from build123d import *

# Parameters (mm, degrees)
ESQUISSE1_W             = 190
ESQUISSE1_H             = 20
BOSS_EXTRU_1_DEPTH      = 6
ESQUISSE2_W             = 6
ESQUISSE2_H             = 20
ENL_V_MAT_EXTRU_1_DEPTH = 3
ESQUISSE3_R             = 1.5
ENL_V_MAT_EXTRU_2_DEPTH = 6


with BuildPart() as part:
    # Esquisse1 → Boss.-Extru.1 (new body)
    with BuildSketch(Plane.XY):
        Rectangle(ESQUISSE1_W, ESQUISSE1_H)
    extrude(amount=BOSS_EXTRU_1_DEPTH)

    # Esquisse2 → Enlèv. mat.-Extru.1 (cut)
    with BuildSketch(Plane.XY.offset(6)):
        with Locations((-92, 0)):
            Rectangle(ESQUISSE2_W, ESQUISSE2_H)
        with Locations((92, 0)):
            Rectangle(ESQUISSE2_W, ESQUISSE2_H)
    extrude(amount=-ENL_V_MAT_EXTRU_1_DEPTH, mode=Mode.SUBTRACT)

    # Esquisse3 → Enlèv. mat.-Extru.2 (cut)
    with BuildSketch(Plane(origin=(0, 0, 0), x_dir=(-1, 0, 0), z_dir=(0, 0, -1))):
        with Locations((-92, -7)):
            Circle(ESQUISSE3_R)
        with Locations((-92, 7)):
            Circle(ESQUISSE3_R)
        with Locations(Location((92, 7, 0), (0, 0, 180))):
            Circle(ESQUISSE3_R)
        with Locations(Location((92, -7, 0), (0, 0, 180))):
            Circle(ESQUISSE3_R)
    extrude(amount=-ENL_V_MAT_EXTRU_2_DEPTH, mode=Mode.SUBTRACT)


solid = part.part
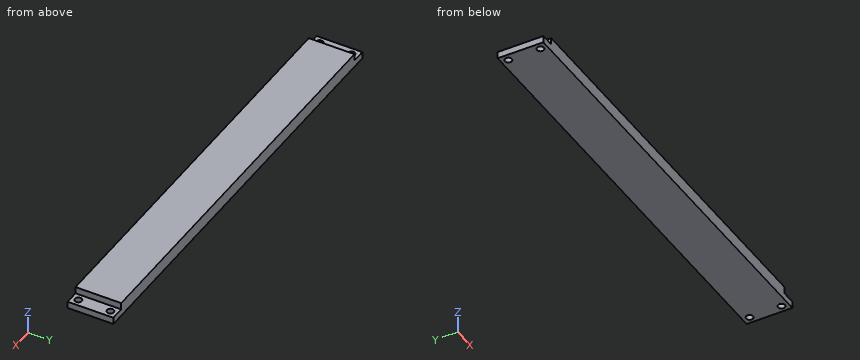
Could you check a few things on this model? Use its own coordinates, in mm. Give positions to 0.01 mm unless a question says otherwise; leave off trailing zeros. Order: outer loops, then holes, each group sorted by start corner. A loop starts at its lowest first (then second) coordinate and runs counter-clockwise, first axis right, second up.
Item 1: If we section it at B-B, the plane z = 4.8: Write out the boundary of the cut face in (x, y).
Item 2: I'm going to push flat-ended pins straight in: pin 1 (2.5 mm diameter, centred on y = 2, z = 4.5, fed in from -X); pin 2 (6.5 mm diameter, centred on x = -93, y = -4.5, fed in from +Z); pin 3 (0.9 mm diameter, centred on y = -2.5, z = 5, fed in from +X). Where does each tip first touch, or does it pass through?
Item 3: I need wall thicknesses on line 1 (Y direction, x = -92, z = 1); line 2 (X direction, y = -5, z = 3.7). Which ranges of each line are inside material? Lowest first, please.
Item 4: If we section it at A-A, the plane y = -2.25: Write out the boundary of the cut face in (x, z).
Values:
1. outline: (-89, -10) - (89, -10) - (89, 10) - (-89, 10) - close
2. pin 1: stops at x = -89
2. pin 2: stops at z = 3
2. pin 3: stops at x = 89
3. line 1: y = -10 to -8.5, -5.5 to 5.5, 8.5 to 10
3. line 2: x = -89 to 89
4. outline: (-95, 0) - (95, 0) - (95, 3) - (89, 3) - (89, 6) - (-89, 6) - (-89, 3) - (-95, 3) - close
